Read the model definition and answer for the solid it produces. Units are mm, in the model's axes. Round coordinates to 2 decimals unless told otherwise and drop trailing zeros. Order: outer loops, then holes, each group sorted by start corner. A loop starts at its lowest first (then second) coordinate and runs counter-clockwise, first axis right, second up. Notation, with made-up numbers: (-16, 0.25) -> (32, 0.25) arc R7 cw to (32, 7.25) -> close; hole circle Ø1 at (37, -32). An arc over 180 degrees is marked (long way). Use a Markdown table: item, result. Add a question column.
1. Consider L1, parallel to Z at x = 0, y = 1.5; L2, parallel to X at y = 6, z = -19; L3, parallel to Z at x = -16, y = 0.5. Determine where each line is inside the solid, lowest interval first. Write a range as [from, to].
2. Given pin 1 (4 mm diameter, centred on x = -18.034, z = 18.034, fed in from -Y); pin 2 (9 mm diameter, centred on x = 0, z = 0, fed in from -Y), each flat-ended and moving along its own axis, determine where each tip first touches the part or whether it passes through.
3. Section D-D, the plane x = -19 is taken. Give the vertices of the cut face in (y, z).
4. Section C-C, the plane y = 1.25 is taken. Give the vertices of the cut face in (x, z).
5. Section B-B, the plane z = -25.4 is taken. Give the vertices of the cut face in (x, y), then the cut area to 3 significant figures.
6. Section A-A, the plane x = 0 is taken. Give the vertices of the cut face in (y, z), then the cut area to 3 significant figures.
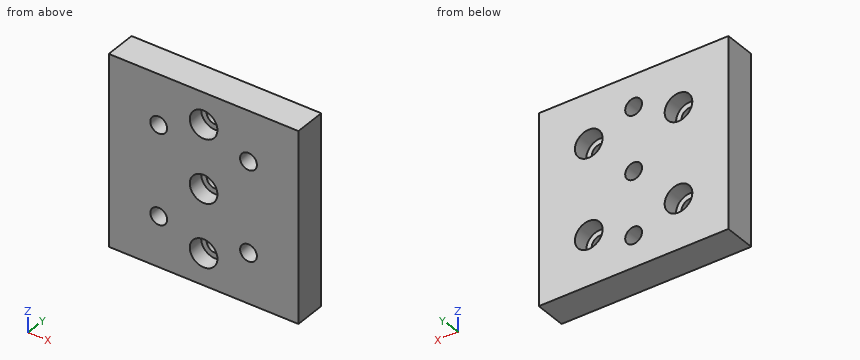
```python
from build123d import *

# Parameters (mm, degrees)
SKETCH1_W                                        = 76.2
SKETCH1_H                                        = 76.2
BOSS_EXTRUDE1_DEPTH                              = 12.7
CBORE_FOR_1_4_SOCKET_HEAD_CAP_SCREW2_D           = 6.7564
CBORE_FOR_1_4_SOCKET_HEAD_CAP_SCREW2_CBORE_D     = 11.1125
CBORE_FOR_1_4_SOCKET_HEAD_CAP_SCREW2_CBORE_DEPTH = 6.35
CBORE_FOR_1_4_SOCKET_HEAD_CAP_SCREW1_D           = 6.7564
CBORE_FOR_1_4_SOCKET_HEAD_CAP_SCREW1_CBORE_D     = 11.1125
CBORE_FOR_1_4_SOCKET_HEAD_CAP_SCREW1_CBORE_DEPTH = 6.35


with BuildPart() as part:
    # Sketch1 → Boss-Extrude1 (new body)
    with BuildSketch(Plane(origin=(0, 0, 0), x_dir=(1, 0, 0), z_dir=(0, 1, 0))):
        Rectangle(SKETCH1_W, SKETCH1_H)
    extrude(amount=BOSS_EXTRUDE1_DEPTH)

    # CBORE for 1/4 Socket Head Cap Screw2 (through all)
    with Locations(Plane(origin=(0, 12.7, 0), x_dir=(1, 0, 0), z_dir=(0, 1, 0))):
        with Locations((-18.034, 18.034), (18.034, 18.034), (18.034, -18.034), (-18.034, -18.034)):
            CounterBoreHole(CBORE_FOR_1_4_SOCKET_HEAD_CAP_SCREW2_D / 2, CBORE_FOR_1_4_SOCKET_HEAD_CAP_SCREW2_CBORE_D / 2, CBORE_FOR_1_4_SOCKET_HEAD_CAP_SCREW2_CBORE_DEPTH)

    # CBORE for 1/4 Socket Head Cap Screw1 (through all)
    with Locations(Plane(origin=(0, 0, 0), x_dir=(-1, 0, 0), z_dir=(0, -1, 0))):
        with Locations((0, 25.4), (0, 0), (0, -25.4)):
            CounterBoreHole(CBORE_FOR_1_4_SOCKET_HEAD_CAP_SCREW1_D / 2, CBORE_FOR_1_4_SOCKET_HEAD_CAP_SCREW1_CBORE_D / 2, CBORE_FOR_1_4_SOCKET_HEAD_CAP_SCREW1_CBORE_DEPTH)


solid = part.part
```
Verdict:
| question | item | result |
|---|---|---|
| 1 | L1 | z = [-38.1, -30.96], [-19.84, -5.56], [5.56, 19.84], [30.96, 38.1] |
| 1 | L2 | x = [-38.1, -21.27], [-14.8, 14.8], [21.27, 38.1] |
| 1 | L3 | z = [-38.1, -20.73], [-15.34, 15.34], [20.73, 38.1] |
| 2 | pin 1 | passes through |
| 2 | pin 2 | stops at y = 6.35 |
| 3 | outline | (0, -38.1) -> (12.7, -38.1) -> (12.7, -23.51) -> (6.35, -23.51) -> (6.35, -21.27) -> (0, -21.27) -> close; (0, -14.8) -> (6.35, -14.8) -> (6.35, -12.56) -> (12.7, -12.56) -> (12.7, 12.56) -> (6.35, 12.56) -> (6.35, 14.8) -> (0, 14.8) -> close; (0, 21.27) -> (6.35, 21.27) -> (6.35, 23.51) -> (12.7, 23.51) -> (12.7, 38.1) -> (0, 38.1) -> close |
| 4 | outline | (-38.1, -38.1) -> (38.1, -38.1) -> (38.1, 38.1) -> (-38.1, 38.1) -> close; hole circle Ø6.76 at (-18.03, -18.03); hole circle Ø6.76 at (-18.03, 18.03); hole circle Ø11.11 at (0, -25.4); hole circle Ø11.11 at (0, 0); hole circle Ø11.11 at (0, 25.4); hole circle Ø6.76 at (18.03, -18.03); hole circle Ø6.76 at (18.03, 18.03) |
| 5 | outline | (-38.1, 0) -> (-5.56, 0) -> (-5.56, 6.35) -> (-3.38, 6.35) -> (-3.38, 12.7) -> (-38.1, 12.7) -> close; (3.38, 6.35) -> (5.56, 6.35) -> (5.56, 0) -> (38.1, 0) -> (38.1, 12.7) -> (3.38, 12.7) -> close |
| 5 | area | 854 mm2 |
| 6 | outline | (0, -38.1) -> (12.7, -38.1) -> (12.7, -28.78) -> (6.35, -28.78) -> (6.35, -30.96) -> (0, -30.96) -> close; (0, -19.84) -> (6.35, -19.84) -> (6.35, -22.02) -> (12.7, -22.02) -> (12.7, -3.38) -> (6.35, -3.38) -> (6.35, -5.56) -> (0, -5.56) -> close; (0, 5.56) -> (6.35, 5.56) -> (6.35, 3.38) -> (12.7, 3.38) -> (12.7, 22.02) -> (6.35, 22.02) -> (6.35, 19.84) -> (0, 19.84) -> close; (0, 30.96) -> (6.35, 30.96) -> (6.35, 28.78) -> (12.7, 28.78) -> (12.7, 38.1) -> (0, 38.1) -> close |
| 6 | area | 627 mm2 |
